from build123d import *

# Parameters (mm, degrees)
SKETCH1_W           = 50
SKETCH1_H           = 6
SKETCH1_W_2         = 6
SKETCH1_H_2         = 50
BOSS_EXTRUDE1_DEPTH = 6


with BuildPart() as part:
    # Sketch1 → Boss-Extrude1 (new body)
    with BuildSketch(Plane(origin=(0, 0, 0), x_dir=(1, 0, 0), z_dir=(0, 1, 0))):
        Polygon((-72, 72), (-72, 28), (-66, 28), (-66, -22), (-72, -22), (-72, -72), (-22, -72), (-22, -66), (28, -66), (28, -72), (72, -72), (72, -22), (72, 28), (72, 72), (28, 72), (-22, 72), align=None)
        with Locations((3, 75)):
            Rectangle(SKETCH1_W, SKETCH1_H)
        with Locations((75, 3)):
            Rectangle(SKETCH1_W_2, SKETCH1_H_2)
    extrude(amount=BOSS_EXTRUDE1_DEPTH)


solid = part.part
CAD build for the part. Positions are in the model's coordinates, mm. A direction names the side the tool comes from. Coordinates: 2 decimals unless noted, no trailing zeros. Loops run counter-clockwise (first coordinate to the right, second up) from the corner with the lowest first, then second, coordinate; pieces in that order, holes last. Notation, with made-up numbers: (34.5, 69.5) -> (48.5, 69.5) arc R19 ccw to (48.5, 83.5) -> close; hole circle Ø6 at (-35.75, 78.5). An arc over 180 degrees is marked (long way). One line per item, written item: value.
1. Slice it at A-A on y = 3.7. Write the cut outline in (x, z), and give its area (3 significant figures).
Answers:
outline: (-72, -72) -> (-22, -72) -> (-22, -78) -> (28, -78) -> (28, -72) -> (72, -72) -> (72, -28) -> (78, -28) -> (78, 22) -> (72, 22) -> (72, 72) -> (28, 72) -> (28, 66) -> (-22, 66) -> (-22, 72) -> (-72, 72) -> (-72, 22) -> (-66, 22) -> (-66, -28) -> (-72, -28) -> close
area: 20,700 mm^2
2. Which spindle directions (+Z, -Z, +X, -X, +Y, -Y) get a long thin tool onto all of the face, cutting with end or side? Do faces 1 (the face through (78, 3, -3)), 2 (the face through (-69, 3, -28)), 3 (the face through (72, 3, -50)), 4 (the face through (-22, 3, -75)), 5 (the face through (-22, 3, 69)). Say none if no direction does.
Answers:
face 1: +Z, -Z, +X, +Y, -Y
face 2: -X, +Y, -Y
face 3: -Z, +X, +Y, -Y
face 4: -Z, -X, +Y, -Y
face 5: +Z, +Y, -Y
3. Pull direction X, two halves, no side cores. Call faces 6 (the face through (72, 3, 47)), 7 (the face through (75, 3, 22)), 8 (the face through (28, 3, 69)): pulls with the +X half, pulls with the -X half, needs draft (parallel to the pull), parting line crosses it, or undercut.
Answers:
face 6: pulls with the +X half
face 7: needs draft
face 8: undercut
4. Flat gauge pins, fed straight in: P1, Ø3, axis at x = 74.5, y = 3, coming from the -Z side; P2, Ø3, axis at x = 30.5, z = 4, coming from the -Y side; P3, Ø3, axis at x = -69.5, y = 2.5, coming from the -Z side; P4, Ø3, axis at x = 76, y = 3, coming from the +Z side. Where does each tip first touch, or does it go through?
Answers:
P1: stops at z = -28
P2: stops at y = 0
P3: stops at z = -72
P4: stops at z = 22
5. Slice it at C-C on x = -46.5. Write the cut outline in (y, z).
Answers:
outline: (0, -72) -> (6, -72) -> (6, 72) -> (0, 72) -> close
6. Slice it at B-B on z = -53. Write the cut outline in (x, y).
Answers:
outline: (-72, 0) -> (72, 0) -> (72, 6) -> (-72, 6) -> close
7. Drill centre lines: line 1 (Z direction, x = 15.5, y = 3.4); line 2 (X direction, y = 2.05, z = 13.5); line 3 (X direction, y = 2.2, z = -70.5). Where is each one in solid material? Low to high. Write a range as [from, to].
Answers:
line 1: z = [-78, 66]
line 2: x = [-66, 78]
line 3: x = [-72, 72]
